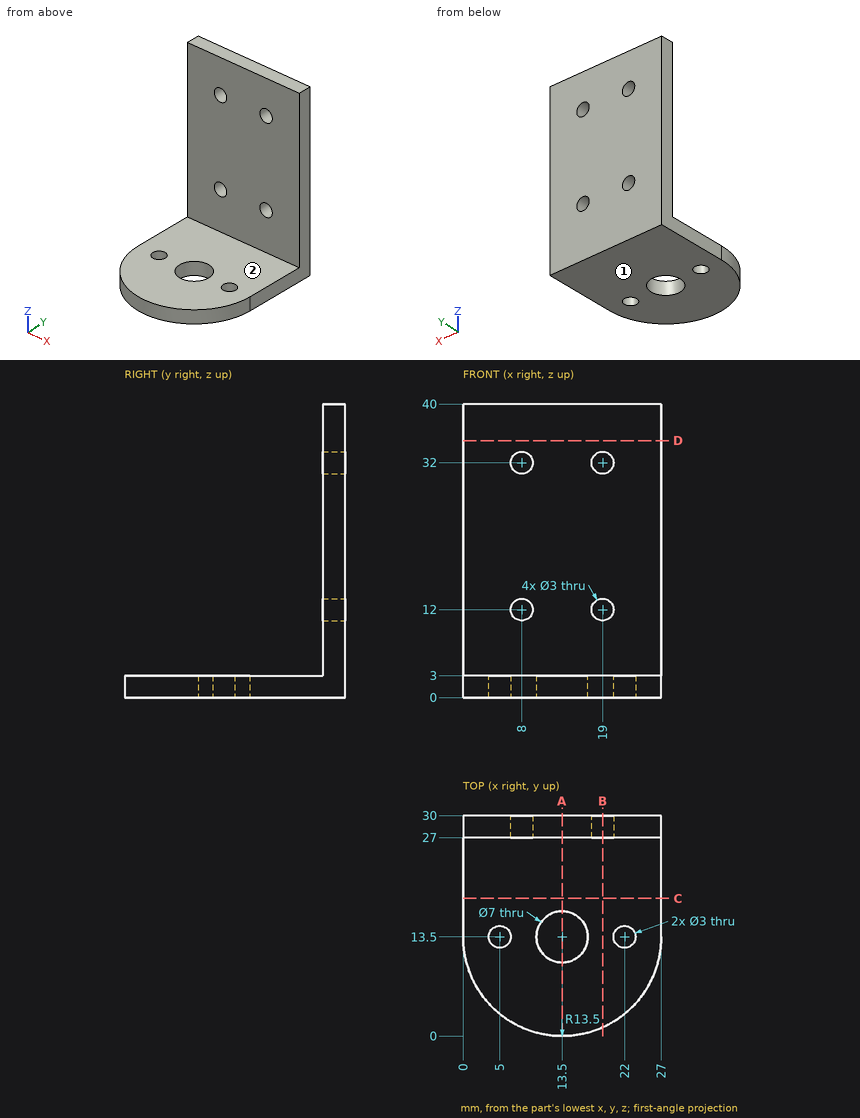
Design review of the part shown in the three views and the two pictorial views. Dimensions are in mm from the part's minimum x, y and z. A direction names the side the tool comes from. Coordinates: 2 decimals unless noted, no trailing zeros. Order: outer loops, then holes, each group sorted by start corner. A loop starts at its lowest first (then second) coordinate and runs counter-clockwise, first axis right, second up.
1) Wall thickness on line 1 along Z through (x, y) = (8, 29.1); line 2 along X through (y, z) = (13.5, 2.3); line 3 along X through (y, z) = (29.4, 12): over which ranges is each line inside the solid? List them lowest first.
2) Clearance check with flat-ended pins moving along their axes: pin 1 (3 mm diameter, centred on x = 9.5, y = 21, fed in from +Z); pin 2 (1.8 mm diameter, centred on x = 8, z = 32, fed in from -Y). State where each tip first meets the part, or that it passes through.
3) Take a section at A-A, the plane x = 13.5. Give the boundary of the cut face in (y, z).
4) Take a section at D-D, the plane z = 35. Give the boundary of the cut face in (x, y).
5) For the marked faces 1 and 2, list the 3-axis set-ups (+Z, -Z, +X, -X, +Y, -Y) from which the entire face can be reached by the end or side of a thin tool; tool diameter is ignored.
6) Take a section at C-C, the plane y = 18.75. Give the boundary of the cut face in (x, z), and give its area (3 significant figures).
7) Take a section at B-B, the plane x = 19. Give the boundary of the cut face in (y, z), and give its area (3 significant figures).
Returned:
1. line 1: z = 0 to 10.5, 13.5 to 30.5, 33.5 to 40
1. line 2: x = 0 to 3.5, 6.5 to 10, 17 to 20.5, 23.5 to 27
1. line 3: x = 0 to 6.5, 9.5 to 17.5, 20.5 to 27
2. pin 1: stops at z = 3
2. pin 2: passes through
3. outline: (0, 0) - (10, 0) - (10, 3) - (0, 3) - close; (17, 0) - (30, 0) - (30, 40) - (27, 40) - (27, 3) - (17, 3) - close
4. outline: (0, 27) - (27, 27) - (27, 30) - (0, 30) - close
5. face 1: -Z, +X, -X, +Y, -Y
5. face 2: +Z, +X, -X, -Y
6. outline: (0, 0) - (27, 0) - (27, 3) - (0, 3) - close
6. area: 81.0 mm2
7. outline: (1.17, 0) - (30, 0) - (30, 10.5) - (27, 10.5) - (27, 3) - (1.17, 3) - close; (27, 13.5) - (30, 13.5) - (30, 30.5) - (27, 30.5) - close; (27, 33.5) - (30, 33.5) - (30, 40) - (27, 40) - close
7. area: 179 mm2
